Study the drawing (mm; zero at the part's minimum x, y, z) and answer. Coordinates: 2 decimals unless noted, no trailing zeros. Loops run counter-clockwise (first coordinate to the right, second up) from the corner with the lowest first, then second, coordinate; pieces in that order, holes last. Notation, with made-up numbers: (40.25, 9) - (64.25, 9) arc R10 cw to (64.25, 18) - close; hole circle Ø2 at (81.25, -9.5). An arc over 180 degrees is marked (long way). Use CSV: the item, a comma, the result in double quotes.
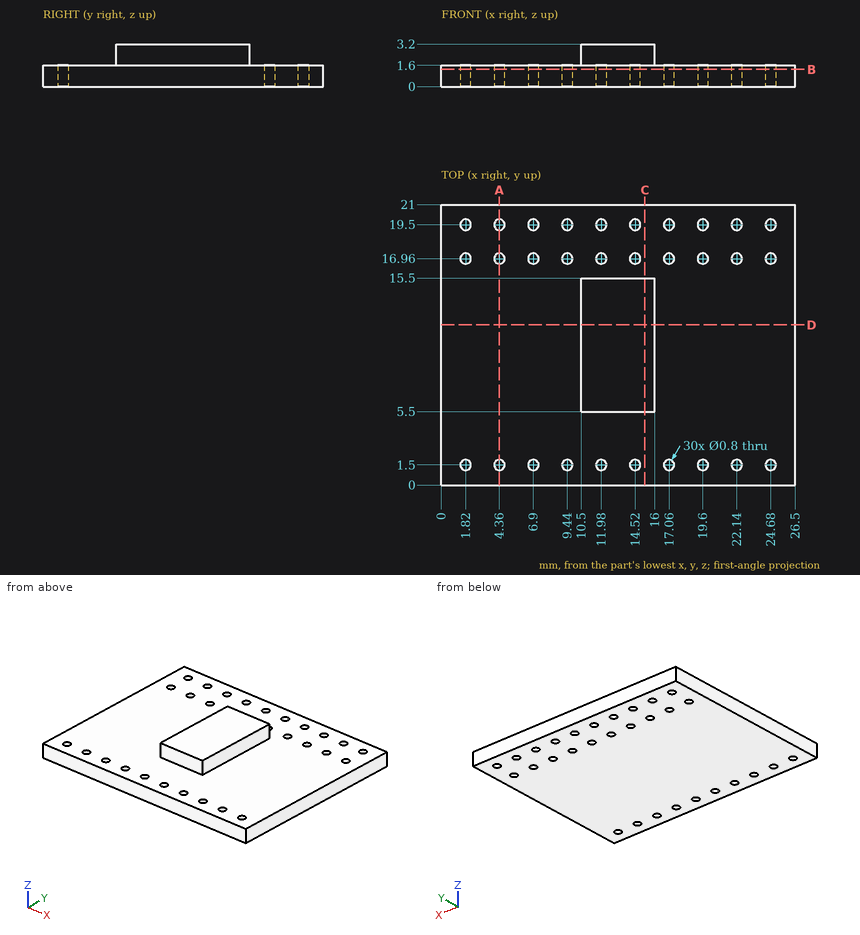
Q1. The part is cut by section A-A on x = 4.36. Determine the outline of the cut face in (y, z).
Reported:
outline,"(0, 0) - (1.1, 0) - (1.1, 1.6) - (0, 1.6) - close; (1.9, 0) - (16.56, 0) - (16.56, 1.6) - (1.9, 1.6) - close; (17.36, 0) - (19.1, 0) - (19.1, 1.6) - (17.36, 1.6) - close; (19.9, 0) - (21, 0) - (21, 1.6) - (19.9, 1.6) - close"
Q2. The part is cut by section B-B on z = 1.3. Give the number of separate pieces and of enclosed holes in the cut face, and give its area (3 significant figures).
Reported:
separate pieces,"1"
enclosed holes,"30"
area,"541 mm²"
Q3. Given P1, Ø3, axis at x = 7.5, y = 16, coming from the +Z side; P2, Ø1.3, axis at y = 11, z = 2.5, coming from the +X side; P3, Ø0.5, axis at y = 12.5, z = 2.5, coming from the -X side, each flat-ended and moving along its own axis, determine where each tip first touches the part or whether it passes through.
Reported:
P1,"stops at z = 1.6"
P2,"stops at x = 16"
P3,"stops at x = 10.5"
Q4. The part is cut by section C-C on x = 15.25. Determine the outline of the cut face in (y, z), and give its area (3 significant figures).
Reported:
outline,"(0, 0) - (21, 0) - (21, 1.6) - (15.5, 1.6) - (15.5, 3.2) - (5.5, 3.2) - (5.5, 1.6) - (0, 1.6) - close"
area,"49.6 mm²"
Q5. Find the intervals of material crossed by probe 1 along Y at (x, z) = (9.44, 1.05); probe 2 along Z at (x, y) = (22.25, 4); probe 3 along Y at (x, z) = (7.25, 0.45), in increasing order. Write a range as [from, to].
Reported:
probe 1,"y = [0, 1.1], [1.9, 16.56], [17.36, 19.1], [19.9, 21]"
probe 2,"z = [0, 1.6]"
probe 3,"y = [0, 1.31], [1.69, 16.77], [17.15, 19.31], [19.69, 21]"
Q6. The part is cut by section D-D on y = 12. Determine the outline of the cut face in (x, z), and give its area (3 significant figures).
Reported:
outline,"(0, 0) - (26.5, 0) - (26.5, 1.6) - (16, 1.6) - (16, 3.2) - (10.5, 3.2) - (10.5, 1.6) - (0, 1.6) - close"
area,"51.2 mm²"
